The model under review builds one solid part; all positions refer to its coordinate system, in mm. A direction names the side the tool comes from. Round coordinates to 2 decimals unless told otherwise and drop trailing zeros. Loops run counter-clockwise (first coordinate to the right, second up) from the corner with the lowest first, then second, coordinate; pieces in that order, holes last. Notation, with made-up numbers: M 43,73 L 77,73 A19 ccw 77,87 Z; hole C 57,81 d2. An arc over 180 degrees is marked long. Answer as a JSON object with one key per item and string values. Group by question number.
Item 1: Consider section B-B (x = 301). Give the boundary of the cut face in (y, z) (3 decimals), and give its area (3 significant figures).
Item 2: Consider section C-C (z = 14.5). Give the boundary of the cut face in (x, y).
Item 3: Consider section A-A (y = -12.7). Give the boundary of the cut face in (x, z).
Item 4: Tool access review of faces 1 (the face through (1295.4, 1, 25)), 2 (the face through (639, -12, 30.55)): name each direction out of +Z, -Z, +X, -X, +Y, -Y from which nothing blocks a thin tool from reaching the whole face with its end or side.
Item 5: The part is to be moulded in two halves that separate along Y. For faces 3 (the face through (0, 1, 25)), 4 (the face through (639, 1.2, 14)), 5 (the face through (639, 0, 14)), say which applies: +Y half, -Y half, draft (parallel to the pull), parting line (faces both ways), or undercut.
Item 6: To check wall thickness, follow line 1 (Z direction, x = 1055, y = -10); line 2 (Y direction, x = 462.5, z = 29.5); line 3 (Y direction, x = 541, z = 3). State the ranges of each line that lie inside material, in increasing order.
Item 7: Insertion check: P1, Ø13, axis at x = 773.4, y = -12.7, coming from the -Z side; P2, Ø8.5, axis at x = 614, z = 17, coming from the -Y side. Each pin has a flat end and moves straight along its axis. Give the tip position at first contact, or say it passes through.
```python
from build123d import *

# Parameters (mm, degrees)
F1_DEPTH = 1295.4
F2_R     = 5
F3_DEPTH = 25.4
F4_R     = 5.08


with BuildPart() as f1:
    # F0 (on Right) → F1 (new body)
    with BuildSketch(Plane.YZ):
        with BuildLine():
            Line((0, 28.518), (0, 0))
            Line((0, 0), (1.2, 0))
            Line((1.2, 0), (1.2, 29.21))
            ThreePointArc((1.2, 29.21), (0.456051, 31.006051), (-1.34, 31.75))
            Line((-1.34, 31.75), (-22.225, 31.75))
            Line((-22.225, 31.75), (-22.225, 30.55))
            Line((-22.225, 30.55), (-2.032, 30.55))
            ThreePointArc((-2.032, 30.55), (-0.595159, 29.954841), (0, 28.518))
        make_face()
    extrude(amount=F1_DEPTH)

    # F2 (on face) → F3 (cut)
    with BuildSketch(Plane.XY.offset(31.75)):
        with Locations((22, -12.7)):
            Circle(F2_R)
        with Locations((272, -12.7)):
            Circle(F2_R)
        with Locations((522, -12.7)):
            Circle(F2_R)
        with Locations((1273.4, -12.7)):
            Circle(F2_R)
        with Locations((1023.4, -12.7)):
            Circle(F2_R)
        with Locations((773.4, -12.7)):
            Circle(F2_R)
    extrude(amount=-F3_DEPTH, mode=Mode.SUBTRACT)

    # F4
    f4_edges = [f1.edges().sort_by_distance(p)[0] for p in [
        (1295.4, 0.6, 0),
        (0, 0.6, 0),
    ]]
    fillet(f4_edges, radius=F4_R)


solid = f1.part
```
Geometry results:
{
 "1": {"outline": "M -22.225,30.55 L -2.032,30.55 A2.032 cw 0,28.518 L 0,0 L 1.2,0 L 1.2,29.21 A2.54 ccw -1.34,31.75 L -22.225,31.75 Z", "area": "64.3 mm^2"},
 "2": {"outline": "M 0,0 L 1295.4,0 L 1295.4,1.2 L 0,1.2 Z"},
 "3": {"outline": "M 0,30.55 L 17,30.55 L 17,31.75 L 0,31.75 Z; M 27,30.55 L 267,30.55 L 267,31.75 L 27,31.75 Z; M 277,30.55 L 517,30.55 L 517,31.75 L 277,31.75 Z; M 527,30.55 L 768.4,30.55 L 768.4,31.75 L 527,31.75 Z; M 778.4,30.55 L 1018.4,30.55 L 1018.4,31.75 L 778.4,31.75 Z; M 1028.4,30.55 L 1268.4,30.55 L 1268.4,31.75 L 1028.4,31.75 Z; M 1278.4,30.55 L 1295.4,30.55 L 1295.4,31.75 L 1278.4,31.75 Z"},
 "4": {"face 1": "+Z, -Z, +X, +Y, -Y", "face 2": "-Z, +X, -X, -Y"},
 "5": {"face 3": "draft", "face 4": "+Y half", "face 5": "-Y half"},
 "6": {"line 1": "z = 30.55 to 31.75", "line 2": "y = -0.25 to 1.18", "line 3": "y = 0 to 1.2"},
 "7": {"P1": "stops at z = 30.55", "P2": "stops at y = 0"}
}
